Autodesk Inventor part; units mm, degrees
ref_plane "YZ Plane" through (0, 0, 0) normal (1, 0, 0) x (0, 1, 0)
ref_plane "XZ Plane" through (0, 0, 0) normal (0, 1, 0) x (-1, 0, 0)
ref_plane "XY Plane" through (0, 0, 0) normal (0, 0, 1) x (1, 0, 0)
sketch "Skizze1" plane through (0, 0, 0) normal (0, 1, 0) x (-1, 0, 0)
  line L0 (1, 0) -> (40, 0)
  line L1 (41, 1) -> (41, 70)
  line L2 (40, 71) -> (1, 71)
  line L3 (0, 70) -> (0, 1)
  line L4 (42.5, 70.5) -> (42.5, 0.5)
  line L5 (40.5, -1.5) -> (0.5, -1.5)
  line L6 (-1.5, 0.5) -> (-1.5, 70.5)
  line L7 (0.5, 72.5) -> (40.5, 72.5)
  arc A0 (42.5, 70.5) -> (40.5, 72.5) centre (40.5, 70.5) ccw
  arc A1 (40.5, -1.5) -> (42.5, 0.5) centre (40.5, 0.5) ccw
  arc A2 (-1.5, 0.5) -> (0.5, -1.5) centre (0.5, 0.5) ccw
  arc A3 (0.5, 72.5) -> (-1.5, 70.5) centre (0.5, 70.5) ccw
  arc A4 (41, 70) -> (40, 71) centre (40, 70) ccw
  arc A5 (40, 0) -> (41, 1) centre (40, 1) ccw
  arc A6 (0, 1) -> (1, 0) centre (1, 1) ccw
  arc A7 (1, 71) -> (0, 70) centre (1, 70) ccw
  point P0 (0, 0)
  point P1 (41, 71)
  point P2 (41, 0)
  point P3 (0, 71)
  dimension "d0" = 41
  dimension "d1" = 71
  dimension "d2" = 1.5
  dimension "d3" = 2
  dimension "d4" = 1
extrude "Extrusion1" add sketch "Skizze1" along normal blind 11
sketch "Skizze2" plane through (0, 11, 0) normal (0, 1, 0) x (1, 0, 0)
  line L0 (1.5, -70.5) -> (1.5, -0.5)
  arc A0 (1.5, -0.5) -> (-0.5, 1.5) centre (-0.5, -0.5) ccw
  line L1 (-0.5, 1.5) -> (-40.5, 1.5)
  arc A1 (-40.5, 1.5) -> (-42.5, -0.5) centre (-40.5, -0.5) ccw
  line L2 (-42.5, -0.5) -> (-42.5, -70.5)
  arc A2 (-42.5, -70.5) -> (-40.5, -72.5) centre (-40.5, -70.5) ccw
  line L3 (-40.5, -72.5) -> (-0.5, -72.5)
  arc A3 (-0.5, -72.5) -> (1.5, -70.5) centre (-0.5, -70.5) ccw
  arc A4 (0, -1) -> (-1, 0) centre (-1, -1) ccw
  line L4 (0, -1) -> (0, -70)
  arc A5 (-1, -71) -> (0, -70) centre (-1, -70) ccw
  line L5 (-1, -71) -> (-40, -71)
  arc A6 (-41, -70) -> (-40, -71) centre (-40, -70) ccw
  line L6 (-41, -70) -> (-41, -1)
  arc A7 (-40, 0) -> (-41, -1) centre (-40, -1) ccw
  line L7 (-40, 0) -> (-1, 0)
  point P0 (0, 0)
extrude "Extrusion2" add sketch "Skizze2" along normal blind 1 contours A3 L3 A2 L2 A1 L1 A0 L0 | L4 A5 L5 A6 L6 A7 L7 A4
fillet "Rundung1" radius 1 8 edges at (0.9142, 12, -0.9142) (-20.5, 12, -1.5) (-41.9142, 12, -0.9142) (-42.5, 12, 35.5) (-41.9142, 12, 71.9142) (-20.5, 12, 72.5) (0.9142, 12, 71.9142) (1.5, 12, 35.5)
sketch "Skizze5" plane through (0, 12, 0) normal (0, 1, 0) x (1, 0, 0)
  line L0 (-34, -65) -> (-9, -65)
  line L1 (-9, -65) -> (-9, -16)
  line L2 (-9, -16) -> (-34, -16)
  line L3 (-34, -16) -> (-34, -65)
  line L4 (-40, 0) -> (-1, 0)
  line L5 (-41, -70) -> (-41, -1)
  line L6 (0, -1) -> (0, -70)
  point P0 (0, 0)
  dimension "d22" = 16
  dimension "d23" = 7
  dimension "d24" = 9
  dimension "d25" = 49
extrude "Extrusion5" cut sketch "Skizze5" against normal blind 10
sketch "Skizze6" plane through (-0.5, 0, -1.5) normal (0, 0, -1) x (-1, 0, 0)
  line L0 (39.5, 0) -> (0.5, 0)
  line L1 (25, 0) -> (15, 0)
  line L2 (15, 0) -> (15, 8)
  line L3 (15, 8) -> (25, 8)
  line L4 (25, 8) -> (25, 0)
  line L5 (42, 0) -> (42, 11)
  point P0 (-0.5, 0)
  dimension "d28" = 8
  dimension "d29" = 10
  dimension "d30" = 17
extrude "Extrusion6" cut sketch "Skizze6" against normal blind 11
properties part number "wanne"
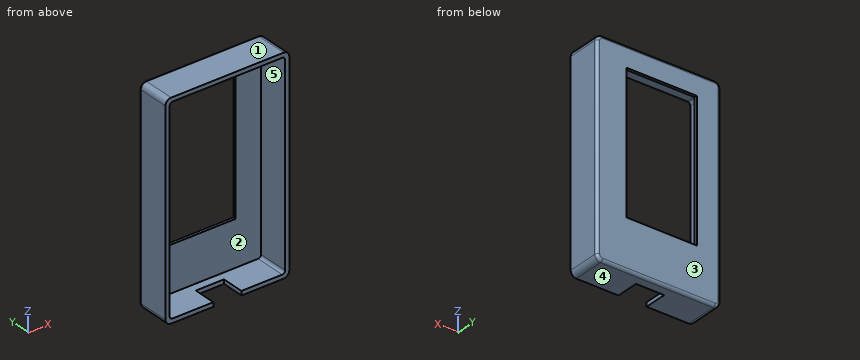
Build history of the part. All positions in model axes, mm. Face numbers are marked on the shaded views. A direction names the side the tool comes from. Round coordinates to 2 decimals unless told otherwise and drop trailing zeros. Write each loop counter-clockwise with the first axis right and the second up, starting at its lowest first coordinate (ties: lowest second). Pieces come first, ordered by that corner, then holes. Notation, with made-up numbers: (17, 51) -> (61, 51) arc R26 cw to (61, 78) -> close; hole circle Ø8 at (7, -13.75). An arc over 180 degrees is marked (long way). Put each result on its own line as item: value.
Item 1: Slice it at C-C, the plane z = 60. Give the cut face in (x, y).
Here are the results:
outline: (-42.5, 0) -> (-41, 0) -> (-41, 11) -> (-34, 11) -> (-34, 12) -> (-41.5, 12) arc R1 ccw to (-42.5, 11) -> close; (-9, 11) -> (0, 11) -> (0, 0) -> (1.5, 0) -> (1.5, 11) arc R1 ccw to (0.5, 12) -> (-9, 12) -> close
Item 2: Flat gauge pins, fed straight in: P1, Ø1.1, axis at x = -27, y = 11.5, coming from the +Z side; P2, Ø0.8, axis at x = -20, z = -0.5, coming from the -Y side; P3, Ø12.5, axis at x = -15, z = 41.5, coming from the -Y side; P4, Ø0.8, axis at y = 11.5, z = 30.5, coming from the -X side (3 decimals). Where does each tip first touch, or does it go through?
Here are the results:
P1: stops at z = 72.5
P2: stops at y = 8
P3: stops at y = 11
P4: stops at x = -42.495
Item 3: Slice it at A-A, the plane x = -26.5. Give the cut face in (y, z), plus the area to 3 significant figures.
Here are the results:
outline: (0, -1.5) -> (11, -1.5) arc R1 ccw to (12, -0.5) -> (12, 16) -> (11, 16) -> (11, 0) -> (0, 0) -> close; (0, 71) -> (11, 71) -> (11, 65) -> (12, 65) -> (12, 71.5) arc R1 ccw to (11, 72.5) -> (0, 72.5) -> close
area: 57.6 mm^2
Item 4: Wall check: probe 1 along X at (y, z) = (8.5, 46); probe 2 along Z at (x, y) = (-23, 9); probe 3 along Y at (x, z) = (-17, 8.5). Give the ranges that are in metal, low to high. Write a range as from..to.
Here are the results:
probe 1: x = -42.5..-41, 0..1.5
probe 2: z = -1.5..0, 71..72.5
probe 3: y = 11..12
Item 5: Tool access for the marked faces 4 and 5: list every direction of +Z, -Z, +X, -X, +Y, -Y with a clear straight run to the whole face (end or side of a thin tool).
Here are the results:
face 4: -Z, +X, -X, +Y, -Y
face 5: -Y
Item 6: Slice it at D-D, the plane y = 2.5. Give the cut face in (x, z), plus the area to 3 significant figures.
Here are the results:
outline: (-42.5, 0.5) arc R2 ccw to (-40.5, -1.5) -> (-25.5, -1.5) -> (-25.5, 0) -> (-40, 0) arc R1 cw to (-41, 1) -> (-41, 70) arc R1 cw to (-40, 71) -> (-1, 71) arc R1 cw to (0, 70) -> (0, 1) arc R1 cw to (-1, 0) -> (-15.5, 0) -> (-15.5, -1.5) -> (-0.5, -1.5) arc R2 ccw to (1.5, 0.5) -> (1.5, 70.5) arc R2 ccw to (-0.5, 72.5) -> (-40.5, 72.5) arc R2 ccw to (-42.5, 70.5) -> close
area: 327 mm^2
Item 7: Slice it at B-B, the plane y = 9. Give the cut face in (x, z).
Here are the results:
outline: (-42.5, 0.5) arc R2 ccw to (-40.5, -1.5) -> (-0.5, -1.5) arc R2 ccw to (1.5, 0.5) -> (1.5, 70.5) arc R2 ccw to (-0.5, 72.5) -> (-40.5, 72.5) arc R2 ccw to (-42.5, 70.5) -> close; hole (-41, 1) arc R1 ccw to (-40, 0) -> (-1, 0) arc R1 ccw to (0, 1) -> (0, 70) arc R1 ccw to (-1, 71) -> (-40, 71) arc R1 ccw to (-41, 70) -> close
Item 8: Two-plate mould, pull along Z, no slides. Class the marked faces 1, 2 and 3: pulls with the +Z half, pulls with the -Z half, needs draft (parallel to the pull), parting line crosses it, or undercut.
Here are the results:
face 1: pulls with the +Z half
face 2: undercut
face 3: needs draft
